```python
from build123d import *

# Parameters (mm, degrees)
F1_DEPTH = 25


with BuildPart() as f1:
    # F0 (on Right) → F1 (new body)
    with BuildSketch(Plane.YZ):
        with BuildLine():
            Line((0, 21), (0, 24))
            ThreePointArc((0, 24), (-16.970563, 16.970563), (-24, 0))
            Line((-24, 0), (-21, 0))
            ThreePointArc((-21, 0), (-14.849242, 14.849242), (0, 21))
        make_face()
        with BuildLine():
            Line((-21, 0), (-24, 0))
            ThreePointArc((-24, 0), (-21.194852, -11.259585), (-13.435146, -19.887103))
            Line((-13.435146, -19.887103), (-11.755753, -17.401215))
            ThreePointArc((-11.755753, -17.401215), (-18.545496, -9.852137), (-21, 0))
        make_face()
        with BuildLine():
            Line((21, 0), (24, 0))
            ThreePointArc((24, 0), (16.970563, 16.970563), (0, 24))
            Line((0, 24), (0, 21))
            ThreePointArc((0, 21), (14.849242, 14.849242), (21, 0))
        make_face()
        with BuildLine():
            Line((12.928941, -16.548187), (14.775932, -18.912213))
            ThreePointArc((14.775932, -18.912213), (21.571073, -10.520875), (24, 0))
            Line((24, 0), (21, 0))
            ThreePointArc((21, 0), (18.874689, -9.205766), (12.928941, -16.548187))
        make_face()
    extrude(amount=F1_DEPTH)


solid = f1.part
```
Design review of the part built by this model. Coordinates are the model's own, in mm. A direction names the side the tool comes from. Give positions to 0.01 mm unless a question says otherwise; leave off trailing zeros. Order: outer loops, then holes, each group sorted by start corner. A loop starts at its lowest first (then second) coordinate and runs counter-clockwise, first axis right, second up. Notation, with made-up numbers: (-23, 8.25) - (-12, 8.25) arc R8 ccw to (-12, 13.25) - close; hole circle Ø11 at (4.5, -24). An arc over 180 degrees is marked (long way). Use a Markdown table: item, result. Add a question column.
(1) Add section D-D on y = -2.5. Give the boundary of the cut face in (x, z), then the cut area to 3 significant figures.
(2) Add section B-B on z = -14. Give the boundary of the cut face in (x, y), then the cut area to 3 significant figures.
(3) Machinability: for faces 1 (the face through (25, -7, 20)), 2 (the face through (12.325, -12.607, -18.662)), which of the approach directions +Z, -Z, +X, -X, +Y, -Y give a long, thin tool a straight path to every point of the face, cutting with its end or side? Answer none if there is none.
(4) Mouldability with a two-part tool opening along Y and no side actions: class faces 3 (the face through (0, -7, 20)), 4 (the face through (12.325, 13.84, -17.714)) as +Y half, -Y half, draft (parallel to the pull), parting line (faces both ways), or undercut.
(5) Wall thickness on probe 1 along Y at (x, z) = (19.5, 8.5); probe 2 along Y at (x, z) = (19.75, 1.5); probe 3 along Z at (x, y) = (10.5, -13): over which ranges is each line inside the solid? List them lowest first. Write a range as [from, to].
(6) Add section C-C on y = -17.5. Give the boundary of the cut face in (x, z), then the cut area to 3 significant figures.
(7) Clearance check with flat-ended pins moving along their axes: P1, Ø2, axis at x = 12, z = 4.5, coming from the -Y side; P2, Ø6, axis at x = 16.5, y = 18, coming from the +Z side (3 decimals); P3, Ø1, axis at x = 21, y = 9.5, coming from the +Z side. State where each tip first meets the part, or that it passes through.
(8) Add section A-A on x = 19.75. Give the boundary of the cut face in (y, z), then the cut area to 3 significant figures.
Report:
| question | item | result |
|---|---|---|
| 1 | outline | (0, 20.85) - (25, 20.85) - (25, 23.87) - (0, 23.87) - close |
| 1 | area | 75.5 mm² |
| 2 | outline | (0, -19.49) - (25, -19.49) - (25, -15.65) - (0, -15.65) - close; (0, 15.65) - (25, 15.65) - (25, 19.49) - (0, 19.49) - close |
| 2 | area | 192 mm² |
| 3 | face 1 | +Z, -Z, +X, +Y, -Y |
| 3 | face 2 | -Z, +X, -X |
| 4 | face 3 | draft |
| 4 | face 4 | undercut |
| 5 | probe 1 | y = [-22.44, -19.2], [19.2, 22.44] |
| 5 | probe 2 | y = [-23.95, -20.95], [20.95, 23.95] |
| 5 | probe 3 | z = [-19.24, -16.49], [16.49, 20.17] |
| 6 | outline | (0, -16.42) - (25, -16.42) - (25, -11.61) - (0, -11.61) - close; (0, 11.61) - (25, 11.61) - (25, 16.42) - (0, 16.42) - close |
| 6 | area | 241 mm² |
| 7 | P1 | stops at y = -23.74 |
| 7 | P2 | stops at z = 18.735 |
| 7 | P3 | stops at z = 22.25 |
| 8 | outline | (-24, 0) arc R24 ccw to (-13.44, -19.89) - (-11.76, -17.4) arc R21 cw to (-21, 0) arc R21 cw to (0, 21) arc R21 cw to (21, 0) arc R21 cw to (12.93, -16.55) - (14.78, -18.91) arc R24 ccw to (24, 0) arc R24 ccw to (0, 24) arc R24 ccw to start |
| 8 | area | 339 mm² |
